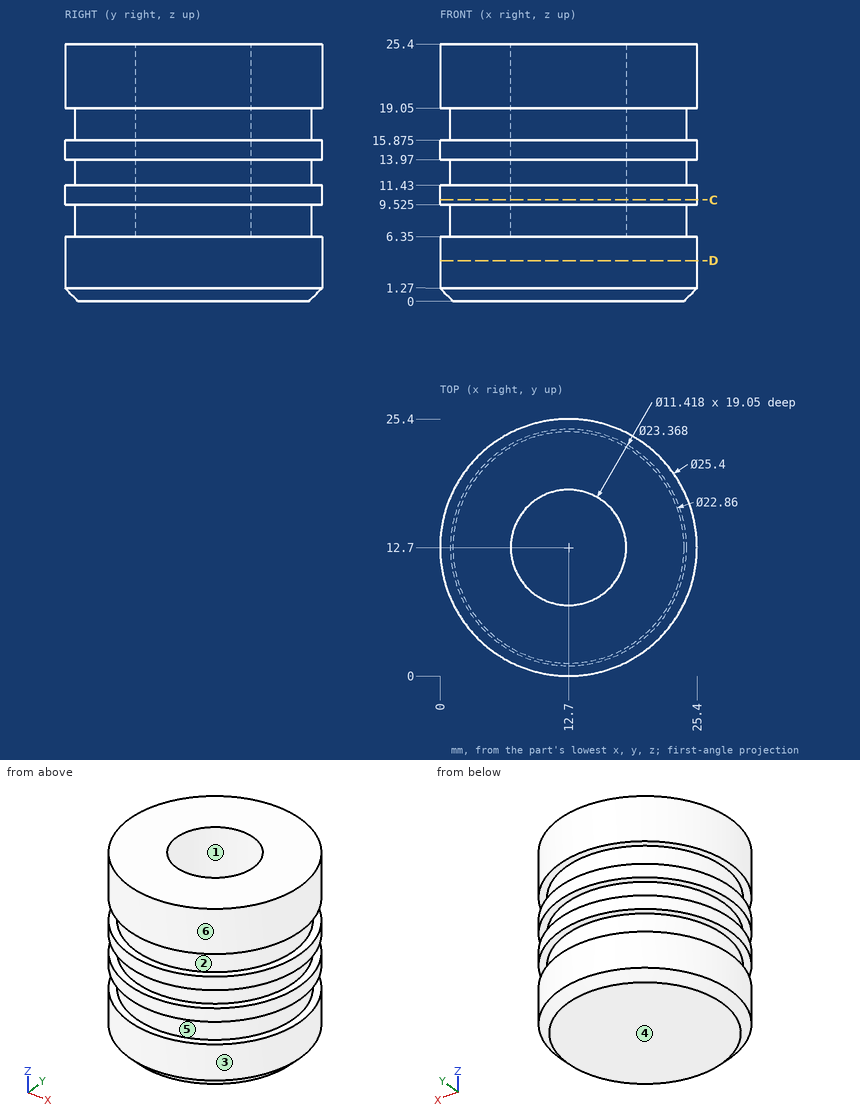
Print and shaded views of the part. All mm, measured from the part's lowest x, y and z. A direction names the side the tool comes from. Give positions to 0.01 mm unless a question says otherwise; leave off trailing zeros. Order: outer loops, then holes, each group sorted by start corner. A loop starts at its lowest first (then second) coordinate and runs counter-clockwise, first axis right, second up. Notation, with made-up numbers: (-25, 16.5) -> (4, 16.5) arc R21 cw to (4, 35.5) -> close; hole circle Ø6 at (57.25, 77). An arc over 180 degrees is marked (long way). Use CSV: the item, a comma, the result in double quotes.
1. Mould opens along Z. For the marked faces 4, 5 and 6 say: +Z half, -Z half, draft (parallel to the pull), parting line (faces both ways), or undercut.
Outcome:
face 4,"-Z half"
face 5,"undercut"
face 6,"draft"
2. Band-saw the part on C-C, the plane z = 10. Give the cut face in (x, y), then the cut area to 3 significant figures.
Outcome:
outline,"circle Ø25.4 at (12.7, 12.7); hole circle Ø11.42 at (12.7, 12.7)"
area,"404 mm²"
3. Drill centre lines: line 1 along Y through (x, z) = (12.7, 14); line 2 along Z through (x, y) = (11, 8.25); line 3 along Y through (x, z) = (12.7, 16.5). Where is each one in solid material? Low to high. Write a range as from..to.
Outcome:
line 1,"0..6.99, 18.41..25.4"
line 2,"0..6.35"
line 3,"1.02..6.99, 18.41..24.38"
4. Drop flat-ended pins along their axis: pin 1 (1 mm diameter, centred on x = 5.5, z = 4.5, fed in from +Y); pin 2 (6 mm diameter, centred on y = 7, z = 2.5, fed in from +X); pin 3 (4 mm diameter, centred on x = 15, z = 6.5, fed in from -Y). Give the stop position or say it passes through.
Outcome:
pin 1,"y = 23.49"
pin 2,"x = 25.11"
pin 3,"y = 0"
5. Band-saw the part on D-D, the plane z = 4. Give the cut face in (x, y), then the cut area to 3 significant figures.
Outcome:
outline,"circle Ø25.4 at (12.7, 12.7)"
area,"507 mm²"
6. 3-axis set-ups, long thin cutter, end or side, ignore diameter. For the marked faces 1, 2 and 3: which of +Z, -Z, +X, -X, +Y, -Y reach the whole face in a straight line?
Outcome:
face 1,"+Z"
face 2,"none"
face 3,"+Z, -Z"
